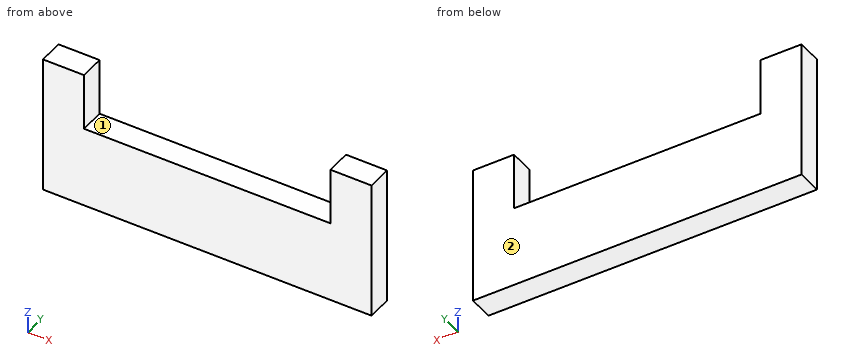
Autodesk Fusion 360 part; units mm, degrees
sketch "Sketch1" plane through (0, 0, 0) normal (0, 0, 1) x (1, 0, 0)
  line L0 (-75, 25) -> (-35, 25)
  line L1 (-35, 25) -> (-35, 20)
  line L2 (-35, 20) -> (-75, 20)
  line L3 (-75, 20) -> (-75, 25)
  line L4 (-75, 20) -> (-70, 20)
  line L5 (-70, 20) -> (-70, 25)
  line L6 (-70, 25) -> (-75, 25)
  line L7 (-75, 25) -> (-75, 20)
  line L8 (-40, 20) -> (-35, 20)
  line L9 (-35, 20) -> (-35, 25)
  line L10 (-35, 25) -> (-40, 25)
  line L11 (-40, 25) -> (-40, 20)
  dimension "d1" = 40
  dimension "d2" = 5
extrude "Extrude1" add sketch "Sketch1" along normal blind 7 contours L0 L2 L3 L4 L5 L6 L7 | L0 L1 L2 L8 L9 L10 L11 makes body 1 at (-70, 21.6667, 2.3333) makes body 2 at (-38.3333, 25, 2.3333)
extrude "Extrude2" add sketch "Sketch1" against normal blind 8 bodies 1 2
extrude "Extrude3" add 1 faces at (-61.6667, 21.6667, -8) along direction (0, 0, -1) blind 2 on bodies 1 bodies 1
extrude "Extrude4" cut 1 faces at (-50, 20, -6.6667) along direction (0, 1, 0) blind 2 on bodies 1 bodies 1
sketch "Sketch2" plane through (0, 25, 0) normal (0, 1, 0) x (-1, 0, 0)
  line L0 (75, -10) -> (75, 7)
  line L1 (75, 7) -> (70, 7)
  line L2 (70, 7) -> (70, 0)
  line L3 (70, 0) -> (40, 0)
  line L4 (40, 0) -> (40, 7)
  line L5 (40, 7) -> (35, 7)
  line L6 (35, 7) -> (35, -10)
  line L7 (35, -10) -> (75, -10)
Work out the finished part from the listing and answer in its coordinate system (mm). Face numbers are marked on the shaded views. Round coordinates to 2 decimals unless told otherwise and drop trailing zeros. Write each loop counter-clockwise with the first axis right and the second up, starting at its lowest first coordinate (ties: lowest second). Pieces come first, ordered by that corner, then holes. Notation, with made-up numbers: M 33,-4.75 L 92,-4.75 A20 cw 92,25.25 Z; hole C -4,-5.5 d10. An arc over 180 degrees is marked long. Use a Markdown table: item, result.
1) The part is cut by section A-A on y = 22.55. Give the vertices of the cut face in (x, z), plus the area to 3 significant figures.
Taken from the geometry:
| item | result |
|---|---|
| outline | M -75,-10 L -35,-10 L -35,7 L -40,7 L -40,0 L -70,0 L -70,7 L -75,7 Z |
| area | 470 mm2 |
2) The part is cut by section B-B on x = -40.5. Give the vertices of the cut face in (y, z).
Taken from the geometry:
| item | result |
|---|---|
| outline | M 22,-10 L 25,-10 L 25,0 L 22,0 Z |
3) Determine the mould class of the marked faces 1 and 2 for opening direction X: pulls with the +X half, pulls with the -X half, needs draft (parallel to the pull), parting line crosses it, or undercut.
Taken from the geometry:
| item | result |
|---|---|
| face 1 | undercut |
| face 2 | needs draft |
4) Consider line 1 (X direction, y = 24.75, z = 2); line 2 (Z direction, x = -66, y = 23.4). Determine where each line is inside the solid, lowest interval first. Write a range as [from, to].
Taken from the geometry:
| item | result |
|---|---|
| line 1 | x = [-75, -70], [-40, -35] |
| line 2 | z = [-10, 0] |
5) A flat-ended cylindrical pin translates along its axis: pin 1 (1 mm diameter, centred on x = -52.5, y = 24, fed in from +Z). Find the tip coordinate at first contact, or state that the pin passes through.
Taken from the geometry:
| item | result |
|---|---|
| pin 1 | stops at z = 0 |
